Geometry: final body of the model. Coordinates: model frame, mm. A direction names the side the tool comes from. Coordinates: 2 decimals unless noted, no trailing zeros. Order: outer loops, then holes, each group sorted by start corner. A loop starts at its lowest first (then second) coordinate and runs counter-clockwise, first axis right, second up. Notation, with made-up numbers: (37, -19.5) -> (43, -19.5) arc R32 ccw to (43, 11.5) -> close; hole circle Ø11 at (69, 39). An arc over 180 degrees is marked (long way). Use one line per item in the form item = value.
```python
from build123d import *

# Parameters (mm, degrees)
SKETCH1_W           = 1500
SKETCH1_H           = 1500
BOSS_EXTRUDE1_DEPTH = 600
CUT_EXTRUDE1_REACH  = 1783.151
SKETCH4_W           = 550
SKETCH4_H           = 300
SKETCH5_W           = 1400
SKETCH5_H           = 500
CUT_EXTRUDE2_DEPTH  = 1150
SKETCH6_W           = 500
SKETCH6_H           = 1100
CUT_EXTRUDE3_DEPTH  = 2364
SKETCH7_W           = 1400
SKETCH7_H           = 1100
CUT_EXTRUDE4_DEPTH  = 320


with BuildPart() as part:
    # Sketch1 → Boss-Extrude1 (new body)
    with BuildSketch(Plane.XY):
        Rectangle(SKETCH1_W, SKETCH1_H)
    extrude(amount=BOSS_EXTRUDE1_DEPTH)

    # Sketch4 → Cut-Extrude1 (cut, up to next)
    with BuildSketch(Plane.ZY.offset(750), mode=Mode.PRIVATE) as cut_extrude1_sk1:
        with Locations((325, 600)):
            Rectangle(SKETCH4_W, SKETCH4_H)
    cut_extrude1_tool1 = extrude(cut_extrude1_sk1.sketch, amount=-CUT_EXTRUDE1_REACH, mode=Mode.PRIVATE) & part.part
    add(cut_extrude1_tool1.solids().sort_by_distance((-750, 600, 325))[0], mode=Mode.SUBTRACT)

    # Sketch5 → Cut-Extrude2 (cut)
    with BuildSketch(Plane.XZ.offset(750)):
        with Locations((0, 300)):
            Rectangle(SKETCH5_W, SKETCH5_H)
    extrude(amount=-CUT_EXTRUDE2_DEPTH, mode=Mode.SUBTRACT)

    # Sketch6 → Cut-Extrude3 (cut)
    with BuildSketch(Plane.ZY.offset(750)):
        with Locations((300, -150)):
            Rectangle(SKETCH6_W, SKETCH6_H)
    extrude(amount=-CUT_EXTRUDE3_DEPTH, mode=Mode.SUBTRACT)

    # Sketch7 → Cut-Extrude4 (cut)
    with BuildSketch(Plane.XY.offset(600)):
        with Locations((0, -150)):
            Rectangle(SKETCH7_W, SKETCH7_H)
    extrude(amount=-CUT_EXTRUDE4_DEPTH, mode=Mode.SUBTRACT)


solid = part.part
```
1) Section D-D, the plane y = 506. Output: boundary loops of the cut face in (x, z).
Results found:
outline = (-750, 0) -> (750, 0) -> (750, 50) -> (-750, 50) -> close
2) Section C-C, the plane y = -235.5. Output: boundary loops of the cut face in (x, z), and give its area (3 significant figures).
Results found:
outline = (-750, 0) -> (750, 0) -> (750, 50) -> (-750, 50) -> close; (-750, 550) -> (-700, 550) -> (-700, 600) -> (-750, 600) -> close; (700, 550) -> (750, 550) -> (750, 600) -> (700, 600) -> close
area = 80,000 mm2
3) Section B-B, the plane z = 408. Output: boundary loops of the cut face in (x, y), and give its area (3 significant figures).
Results found:
outline = (-750, -750) -> (-700, -750) -> (-700, -700) -> (-750, -700) -> close; (-750, 400) -> (750, 400) -> (750, 450) -> (-750, 450) -> close; (700, -750) -> (750, -750) -> (750, -700) -> (700, -700) -> close
area = 80,000 mm2
4) Pull-direction query (Y, two-part tool) for faces 6 (the flat face through (-10, 750, 25)), 7 (the flat face through (-700, -725, 296)), 8 (the flat face through (700, -158, 575)), 9 (the flat face through (725, -158, 550)); classes: released by +Y, released by -Y, zero draft, split by the parting line, or undercut.
Results found:
face_6 = released by +Y
face_7 = zero draft
face_8 = undercut
face_9 = undercut
5) Section A-A, the plane x = 405. Output: boundary loops of the cut face in (y, z).
Results found:
outline = (-750, 0) -> (750, 0) -> (750, 50) -> (450, 50) -> (450, 600) -> (400, 600) -> (400, 50) -> (-750, 50) -> close; (-750, 550) -> (-700, 550) -> (-700, 600) -> (-750, 600) -> close
6) Contact query for flat-ended pins moving along their axis: P1, Ø15, axis at x = -713, z = 363.5, coming from the +Y side; P2, Ø4, axis at x = -532.5, z = 475.5, coming from the -Y side; P3, Ø10, axis at x = 141, y = 535.5, coming from the +Z side. Output: stop coordinate, or through.
Results found:
P1 = 450
P2 = 400
P3 = 50
7) Material intervals for probe 1 along Z at (x, y) = (341, -379); probe 2 along Y at (x, z) = (364.5, 220.5), sorted ascending. Write a range as from..to.
Results found:
probe_1 = 0..50
probe_2 = 400..450
8) Access query for faces 1 (the flat face through (-10, -725, 550)), 2 (the flat face through (-700, -158, 575)), 3 (the flat face through (-59, -725, 600)), 4 (the flat face through (-10, 598, 50)), 5 (the flat face through (-725, -700, 296)). Directions: +Z, -Z, +X, -X, +Y, -Y. A direction counts if a zero-diameter tool reaches every point of the face in a straight line with its end or side. Return the directions, or none.
Results found:
face_1 = -Y
face_2 = +Z
face_3 = +Z, +X, -X, +Y, -Y
face_4 = +Z, +X, -X, +Y
face_5 = +X, -X
